Study the drawing (mm; zero at the part's minimum x, y, z) and answer. Coordinates: 2 decimals unless noted, no trailing zeros. Order: outer loops, then holes, each group sorted by start corner. A loop starts at its lowest first (then second) coordinate and runs counter-clockwise, first axis right, second up. Notation, with made-up numbers: M 69.5,84.25 L 105.5,84.25 A26 cw 105.5,116.25 Z; hole C -39.5,79.25 d3. An arc over 180 degrees is marked long. One line per item, written item: value. Start each with the question number.
Q1. The part is cut by section C-C on y = 7.25. Give the vertices of the cut face in (x, z), then the cut area to 3 significant figures.
Q2. The part is cut by section A-A on z = 2.3. Give the vertices of the cut face in (x, y).
Q3. The part is cut by section B-B on x = 16.5. Give the vertices of the cut face in (y, z).
Q4. Straight lines are drawn through the part: line 1 along X through (y, z) = (5.5, 0.7); line 2 along Y through (x, z) = (18, 0.9); line 3 along Y through (x, z) = (16.25, 2.7). For each, find the intervals that lie inside material, in ascending order. Write a range as [from, to].
Q5. Each of these flat-tipped pins is pushed along its axis until it touches: pin 1 Ø1.5 at (y, z) = (3.5, 1.5) entering from +X; pin 2 Ø1 at (x, z) = (19, 1.5) entering from -Y. Where does it stop, or does it pass through?
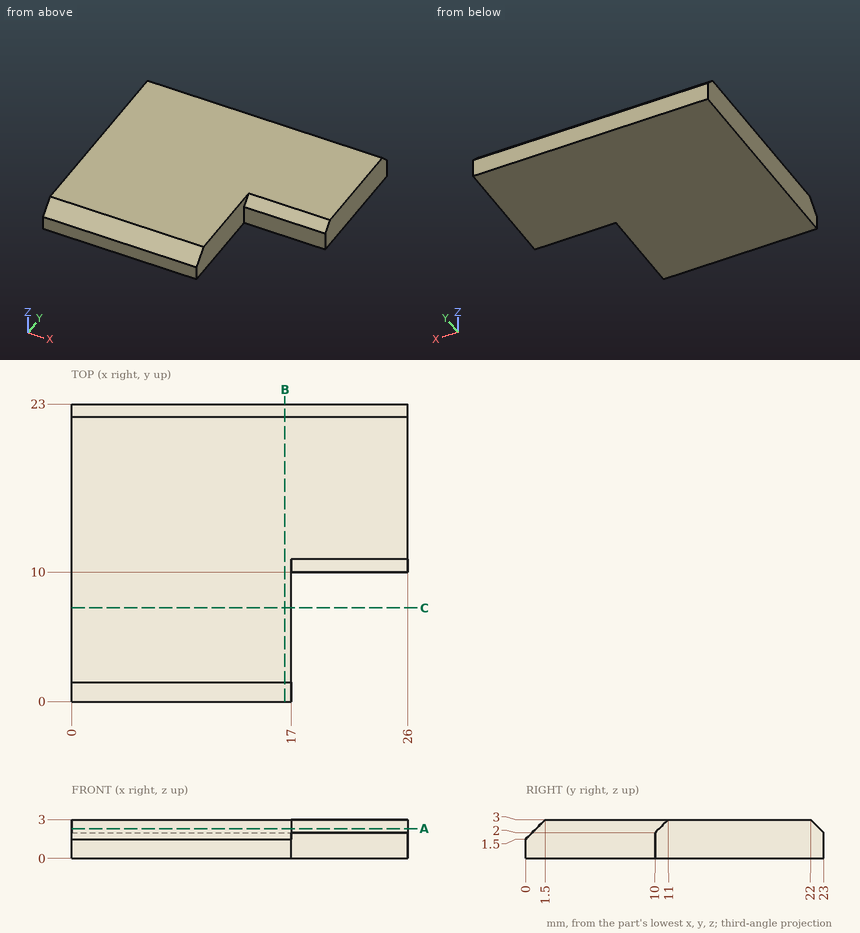
Output:
1. outline: M 0,0 L 17,0 L 17,3 L 0,3 Z
1. area: 51.0 mm^2
2. outline: M 0,0.8 L 17,0.8 L 17,10.3 L 26,10.3 L 26,22.7 L 0,22.7 Z
3. outline: M 0,0 L 23,0 L 23,2 L 22,3 L 1.5,3 L 0,1.5 Z
4. line 1: x = [0, 17]
4. line 2: y = [10, 23]
4. line 3: y = [1.2, 22.3]
5. pin 1: stops at x = 17
5. pin 2: stops at y = 10
